Study the drawing (mm; zero at the part's minimum x, y, z) and answer. A direction names the side the tool comes from. Round coordinates to 2 decimals unless told otherwise and drop trailing zeros. Order: outer loops, then holes, each group sorted by start corner. A loop starts at its lowest first (then second) coordinate and runs counter-clockwise, first axis right, second up. Notation, with made-up numbers: (57.25, 76) -> (83.25, 76) arc R23 ccw to (83.25, 93) -> close; hole circle Ø7 at (-40, -2.75). An arc over 180 degrees is marked (long way). Use one line per item in the form item = value.
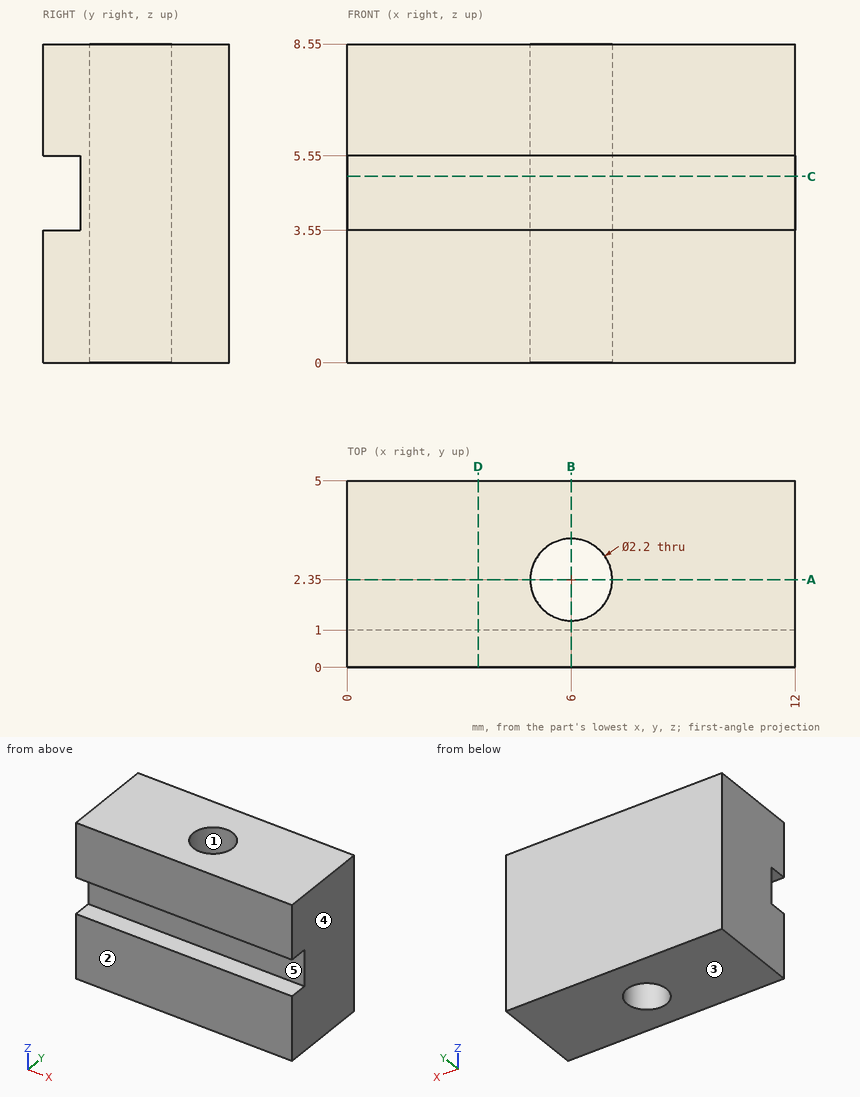
Item 1: The part is cut by section A-A, the plane y = 2.35. Give the vertices of the cut face in (x, z).
Findings:
outline = (0, 0) -> (4.9, 0) -> (4.9, 8.55) -> (0, 8.55) -> close; (7.1, 0) -> (12, 0) -> (12, 8.55) -> (7.1, 8.55) -> close
Item 2: Consider line 1 along X through (y, z) = (2.4, 4); line 2 along Y through (x, z) = (6, 4.5); line 3 along Y through (x, z) = (6, 2). Determine where each line is inside the solid, lowest interval first.
Findings:
line_1 = 0 to 4.9, 7.1 to 12
line_2 = 1 to 1.25, 3.45 to 5
line_3 = 0 to 1.25, 3.45 to 5
Item 3: The part is cut by section C-C, the plane z = 5. Give the vertices of the cut face in (x, y).
Findings:
outline = (0, 1) -> (12, 1) -> (12, 5) -> (0, 5) -> close; hole circle Ø2.2 at (6, 2.35)
Item 4: For the marked faces 4 and 5, determine the directions among +Z, -Z, +X, -X, +Y, -Y from which every point of the face is accessible in a straight line to the end or side of a thin tool.
Findings:
face_4 = +Z, -Z, +X, +Y, -Y
face_5 = +X, -X, -Y
Item 5: The part is cut by section B-B, the plane x = 6. Give the vertices of the cut face in (y, z), and give its area (3 significant figures).
Findings:
outline = (0, 0) -> (1.25, 0) -> (1.25, 8.55) -> (0, 8.55) -> (0, 5.55) -> (1, 5.55) -> (1, 3.55) -> (0, 3.55) -> close; (3.45, 0) -> (5, 0) -> (5, 8.55) -> (3.45, 8.55) -> close
area = 21.9 mm^2
Item 6: The part is cut by section D-D, the plane x = 3.5. Give the vertices of the cut face in (y, z).
Findings:
outline = (0, 0) -> (5, 0) -> (5, 8.55) -> (0, 8.55) -> (0, 5.55) -> (1, 5.55) -> (1, 3.55) -> (0, 3.55) -> close
Item 7: Determine the mould class of the marked faces 1, 2 and 3 for opening direction Y: released by +Y, released by -Y, zero draft, split by the parting line, or undercut.
Findings:
face_1 = undercut
face_2 = released by -Y
face_3 = zero draft
